Can you work these out from the model? Positions are in its coordinate system, mm. Round coordinates to 2 decimals unless told otherwise and drop trailing zeros. Loops run counter-clockwise (first coordinate to the right, second up) from the corner with the lowest first, then second, coordinate; pieces in that order, holes last.
(1) Will these pins go through, and if not, where does the flat tip stop? pin 1 Ø10 at (y, z) = (12, -23) entering from -X; pin 2 Ø2 at (x, z) = (119.5, -47) entering from -Y; pin 3 Ø4 at (x, y) = (162.5, 10) entering from +Z; pin 4 Ø3 at (x, z) = (149, -91.5) entering from +Y.
(2) I want a section at A-A on y = 11.75. Give the number of separate pieces and of enclosed holes in the cut face, plus the area to 3 significant figures.
(3) If I drill on line 1 along X through (y, z) = (1.75, -101.6); line 2 along X through (y, z) = (4.25, -138.5); line 3 along X through (y, z) = (16.25, -78.5), over which ranges is the centre line in solid material (lowest first)?
(4) I want a section at B-B on x = 128. Write out the boundary of the cut face in (y, z).
(5) I want a section at C-C on z = -135. Write out the boundary of the cut face in (x, y), plus the area to 3 significant figures.
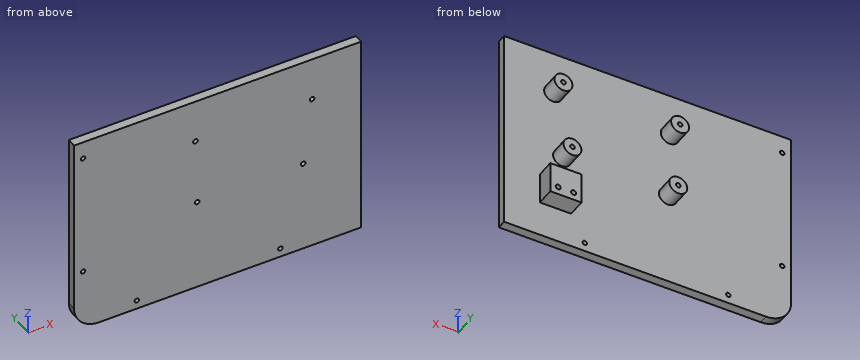
from build123d import *

# Parameters (mm, degrees)
SKETCH1_R           = 1.5875
BOSS_EXTRUDE1_DEPTH = 6.35
SKETCH2_W           = 22.098
SKETCH2_H           = 22.098
SKETCH2_R           = 1.778
BOSS_EXTRUDE2_DEPTH = 12.7
SKETCH3_R           = 6.35
BOSS_EXTRUDE3_DEPTH = 12.7
SKETCH5_R           = 1.651
CUT_EXTRUDE1_DEPTH  = 251.965625136


with BuildPart() as part:
    # Sketch1 → Boss-Extrude1 (new body)
    with BuildSketch(Plane(origin=(0, 0, 0), x_dir=(1, 0, 0), z_dir=(0, 1, 0))):
        with BuildLine():
            Line((0, 0), (203.2, 0))
            Line((203.2, 0), (203.2, 146.05))
            Line((203.2, 146.05), (17.78, 146.05))
            ThreePointArc((17.78, 146.05), (5.207641431, 140.842358569), (0, 128.27))
            Line((0, 128.27), (0, 0))
        make_face()
        with Locations(Location((6.35, 12.7, 0), (0, 0, 270))):
            Circle(SKETCH1_R, mode=Mode.SUBTRACT)
        with Locations(Location((6.35, 101.6, 0), (0, 0, 270))):
            Circle(SKETCH1_R, mode=Mode.SUBTRACT)
        with Locations(Location((44.45, 139.7, 0), (0, 0, 270))):
            Circle(SKETCH1_R, mode=Mode.SUBTRACT)
        with Locations(Location((146.05, 139.7, 0), (0, 0, 270))):
            Circle(SKETCH1_R, mode=Mode.SUBTRACT)
    extrude(amount=BOSS_EXTRUDE1_DEPTH)

    # Sketch2 → Boss-Extrude2 (add)
    with BuildSketch(Plane(origin=(0, 6.35, 0), x_dir=(1, 0, 0), z_dir=(0, 1, 0))):
        with Locations((166.751, 109.601)):
            Rectangle(SKETCH2_W, SKETCH2_H)
        with Locations(Location((172.212, 115.062, 0), (0, 0, 270))):
            Circle(SKETCH2_R, mode=Mode.SUBTRACT)
        with Locations(Location((161.29, 115.062, 0), (0, 0, 270))):
            Circle(SKETCH2_R, mode=Mode.SUBTRACT)
    extrude(amount=BOSS_EXTRUDE2_DEPTH)

    # Sketch3 → Boss-Extrude3 (add)
    with BuildSketch(Plane(origin=(0, 6.35, 0), x_dir=(1, 0, 0), z_dir=(0, 1, 0))):
        with Locations(Location((162.13368637, 79.502, 0), (0, 0, 270))):
            Circle(SKETCH3_R)
        with Locations(Location((168.48368637, 31.242, 0), (0, 0, 270))):
            Circle(SKETCH3_R)
        with Locations(Location((87.20368637, 79.502, 0), (0, 0, 270))):
            Circle(SKETCH3_R)
        with Locations(Location((85.93368637, 31.242, 0), (0, 0, 270))):
            Circle(SKETCH3_R)
    extrude(amount=BOSS_EXTRUDE3_DEPTH)

    # Sketch5 → Cut-Extrude1 (cut, through all)
    with BuildSketch(Plane(origin=(0, 19.05, 0), x_dir=(1, 0, 0), z_dir=(0, 1, 0))):
        with Locations(Location((168.48368637, 31.242, 0), (0, 0, 270))):
            Circle(SKETCH5_R)
        with Locations(Location((162.13368637, 79.502, 0), (0, 0, 270))):
            Circle(SKETCH5_R)
        with Locations(Location((87.20368637, 79.502, 0), (0, 0, 270))):
            Circle(SKETCH5_R)
        with Locations(Location((85.93368637, 31.242, 0), (0, 0, 270))):
            Circle(SKETCH5_R)
    extrude(amount=-CUT_EXTRUDE1_DEPTH, mode=Mode.SUBTRACT)


solid = part.part
Filled sheet:
1. pin 1: stops at x = 80.47
1. pin 2: stops at y = 0
1. pin 3: stops at z = -26.3
1. pin 4: stops at y = 6.35
2. separate pieces: 5
2. enclosed holes: 6
2. area: 941 mm2
3. line 1: x = 0 to 4.76, 7.94 to 203.2
3. line 2: x = 3.24 to 43.41, 45.49 to 145.01, 147.09 to 203.2
3. line 3: x = 80.93 to 85.89, 88.52 to 93.47, 155.86 to 160.82, 163.45 to 168.4
4. outline: (0, -146.05) - (6.35, -146.05) - (6.35, 0) - (0, 0) - close
5. outline: (1.32, 0) - (203.2, 0) - (203.2, 6.35) - (1.32, 6.35) - close
5. area: 1,280 mm2
